Part print with two shaded views. Sizes in mm from the minimum x, y, z corner. Coordinates: 2 decimals unless noted, no trailing zeros. Write each loop counter-clockwise with the first axis right and the second up, starting at its lowest first coordinate (ties: lowest second). Pieces come first, ordered by that corner, then holes. Notation, with made-up numbers: (-24.5, 52.5) - (-5.5, 52.5) arc R20 cw to (-5.5, 91.5) - close; hole circle Ø1 at (-39.75, 52.5). An arc over 180 degrees is marked (long way). Answer in a Markdown table with one row per item. Add a question column.
Q1. Drill centre lines: line 1 along X through (y, z) = (2.4, 180); line 2 along X through (y, z) = (2.1, 30); line 3 along Z through (x, y) = (92.5, 1.2). Where is each one in solid material? Low to high. Write a range as from..to.
Q2. Band-saw the part on B-B (y = 0.95). State how many separate pieces and enclosed holes the cut face has, and give its area (3 significant figures).
Q3. Pin check, flat tips, straight feed: pin 1 (3 mm diameter, centred on x = 7.5, z = 20, fed in from +Y); pin 2 (1 mm diameter, centred on x = 50, y = 2, fed in from -Z); pin 3 (1 mm diameter, centred on x = 43.5, y = 2, fed in from +Z). Stop position of each tip, or through.
Q4. Band-saw the part on A-A (x = 43). List the corners of the cut face in (y, z), and give its area (3 significant figures).
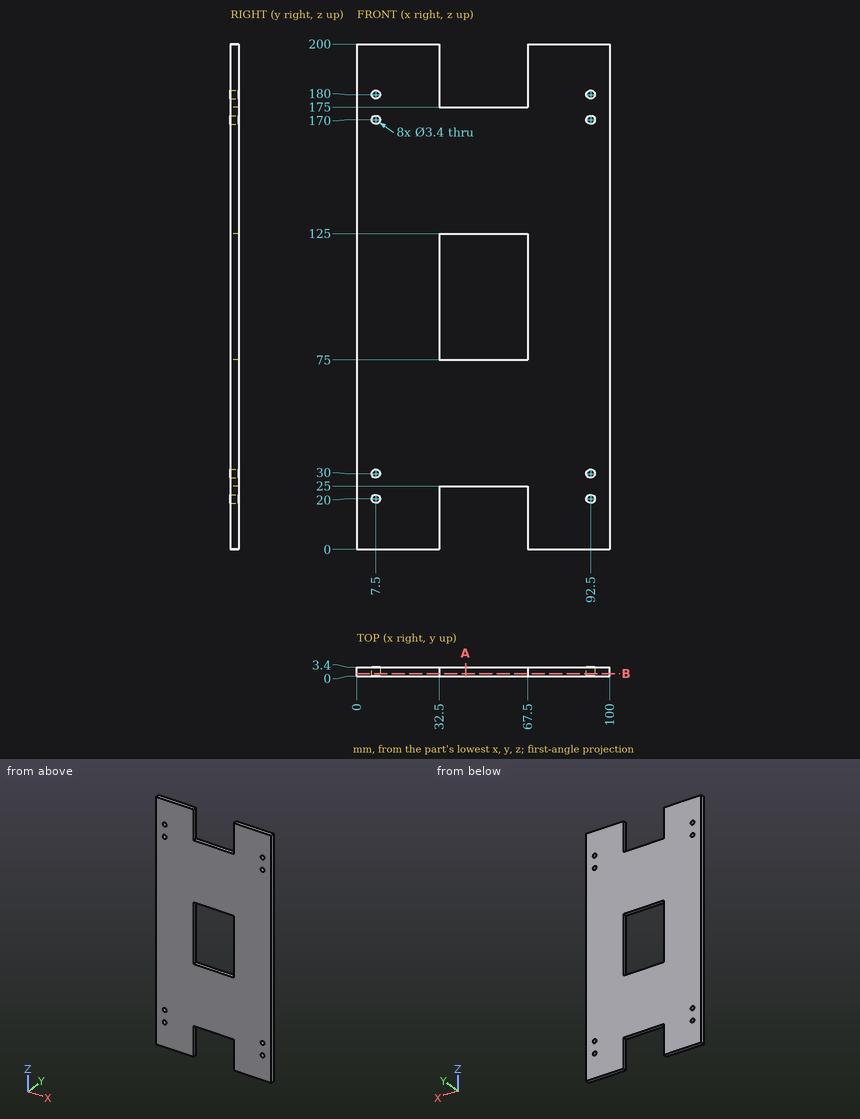
Checked values:
| question | item | result |
|---|---|---|
| 1 | line 1 | x = 0..5.8, 9.2..32.5, 67.5..90.8, 94.2..100 |
| 1 | line 2 | x = 0..5.8, 9.2..90.8, 94.2..100 |
| 1 | line 3 | z = 0..18.3, 21.7..28.3, 31.7..168.3, 171.7..178.3, 181.7..200 |
| 2 | separate pieces | 1 |
| 2 | enclosed holes | 9 |
| 2 | area | 16,400 mm² |
| 3 | pin 1 | passes through |
| 3 | pin 2 | stops at z = 25 |
| 3 | pin 3 | stops at z = 175 |
| 4 | outline | (0, 25) - (3.4, 25) - (3.4, 75) - (0, 75) - close; (0, 125) - (3.4, 125) - (3.4, 175) - (0, 175) - close |
| 4 | area | 340 mm² |
